For this review, take the finished solid that the model builds, in its own axes (mm). A direction names the side the tool comes from. Give positions to 0.01 mm unless a question says otherwise; leave off trailing zeros. Write each loop counter-clockwise with the first axis right and the second up, starting at its lowest first coordinate (ties: lowest second). Pieces come first, ordered by that corner, then holes. Notation, with made-up numbers: (22.25, -37) -> (45.25, -37) arc R15 cw to (45.25, -12) -> close; hole circle Ø7 at (40.25, 83). An arc over 180 degrees is marked (long way). Return JSON: item names as keys, results as strings.
from build123d import *

# Parameters (mm, degrees)
EXTRUDE_1_DEPTH     = 145
SKETCH_2_R          = 2.25
CUT_EXTRUDE_1_DEPTH = 147.626771089


with BuildPart() as part:
    # Эскиз1 → Бобышка-Вытянуть1 (new body)
    with BuildSketch(Plane(origin=(0, 0, 0), x_dir=(1, 0, 0), z_dir=(0, 1, 0))):
        Polygon((0, 0), (10.6, 0), (10.6, 9.5), (15.1, 9.5), (15.1, -5), (-4.5, -5), (-4.5, 9.5), (0, 9.5), align=None)
    extrude(amount=EXTRUDE_1_DEPTH)

    # Эскиз2 → Вырез-Вытянуть1 (cut, through all)
    with BuildSketch(Plane(origin=(15.1, 0, 0), x_dir=(0, 0, -1), z_dir=(1, 0, 0))):
        with Locations((4.5, 40.3)):
            Circle(SKETCH_2_R)
        with Locations((4.5, 8.1)):
            Circle(SKETCH_2_R)
        with Locations((4.5, 72.5)):
            Circle(SKETCH_2_R)
        with Locations((4.5, 104.7)):
            Circle(SKETCH_2_R)
        with Locations((4.5, 136.9)):
            Circle(SKETCH_2_R)
    extrude(amount=-CUT_EXTRUDE_1_DEPTH, mode=Mode.SUBTRACT)


solid = part.part
1. Add section D-D, the plane y = 67.5. State the section outline as (x, z) points.
Results found:
{"outline": "(-4.5, -9.5) -> (0, -9.5) -> (0, 0) -> (10.6, 0) -> (10.6, -9.5) -> (15.1, -9.5) -> (15.1, 5) -> (-4.5, 5) -> close"}
2. To check wall thickness, follow probe 1 along Y at (x, z) = (12.4, -4.5); probe 2 along X at (y, z) = (33.5, -3.5); probe 3 along Z at (x, y) = (1.5, 109). State the ranges of each line that lie inside material, in increasing order.
Results found:
{"probe 1": "y = 0 to 5.85, 10.35 to 38.05, 42.55 to 70.25, 74.75 to 102.45, 106.95 to 134.65, 139.15 to 145", "probe 2": "x = -4.5 to 0, 10.6 to 15.1", "probe 3": "z = 0 to 5"}
3. Add section A-A, the plane y = 40.3. State the section outline as (x, z) points.
Results found:
{"outline": "(-4.5, -9.5) -> (0, -9.5) -> (0, -6.75) -> (-4.5, -6.75) -> close; (-4.5, -2.25) -> (0, -2.25) -> (0, 0) -> (10.6, 0) -> (10.6, -2.25) -> (15.1, -2.25) -> (15.1, 5) -> (-4.5, 5) -> close; (10.6, -9.5) -> (15.1, -9.5) -> (15.1, -6.75) -> (10.6, -6.75) -> close"}
4. Add section C-C, the plane z = -4.5. Count the separate pieces of the cut face and the enclosed holes in it, plus the area to 3 significant figures.
Results found:
{"separate pieces": "12", "enclosed holes": "0", "area": "1,100 mm²"}
5. For pin 1 (3.5 mm diameter, centred on y = 104.7, z = -4.5, fed in from -X), flat-tipped, find the tip position at first contact; note if it passes through.
Results found:
{"pin 1": "passes through"}
6. For faces 5 (the flat face through (-2, 71, -9.5)), 6 (the flat face through (10.6, 71, -7)), list the 3-axis set-ups (+Z, -Z, +X, -X, +Y, -Y) from which the entire face can be reached by the end or side of a thin tool; tool diameter is ignored.
Results found:
{"face 5": "-Z, +X, -X, +Y, -Y", "face 6": "-Z, +Y, -Y"}
7. Add section B-B, the plane x = -2.25. State the section outline as (y, z) points, plus the area to 3 significant figures.
Results found:
{"outline": "(0, -9.5) -> (145, -9.5) -> (145, 5) -> (0, 5) -> close; hole circle Ø4.5 at (8.1, -4.5); hole circle Ø4.5 at (40.3, -4.5); hole circle Ø4.5 at (72.5, -4.5); hole circle Ø4.5 at (104.7, -4.5); hole circle Ø4.5 at (136.9, -4.5)", "area": "2,020 mm²"}
8. The part is to be moulded in two halves that separate along X. For faces 1 (the flat face through (15.1, 71, -2)), 2 (the flat face through (-4.5, 71, -2)), 3 (the flat face through (0, 71, -7)), 4 (the cylindrical face through (-2.219, 70.304, -4.012)), say which applies: +X half, -X half, draft (parallel to the pull), parting line (faces both ways), or undercut.
Results found:
{"face 1": "+X half", "face 2": "-X half", "face 3": "undercut", "face 4": "draft"}
